from build123d import *

# Parameters (mm, degrees)
SKETCH_1_W      = 85
SKETCH_1_H      = 104
SKETCH_1_R      = 2
SKETCH_1_R_2    = 1.5
EXTRUDE_1_DEPTH = 4
FILLET_1_R      = 8


with BuildPart() as part:
    # 草图1 → 凸台-拉伸1 (new body)
    with BuildSketch(Plane.XY):
        with Locations((-13.600288588, -10.520274333)):
            Rectangle(SKETCH_1_W, SKETCH_1_H)
        with Locations((12.899711412, -0.520274333)):
            Circle(SKETCH_1_R, mode=Mode.SUBTRACT)
        with Locations((12.899711412, -20.520274333)):
            Circle(SKETCH_1_R, mode=Mode.SUBTRACT)
        with Locations((-46.100288588, 14.479725667)):
            Circle(SKETCH_1_R, mode=Mode.SUBTRACT)
        with Locations((-46.100288588, -35.520274333)):
            Circle(SKETCH_1_R, mode=Mode.SUBTRACT)
        with Locations((3.899711412, -35.520274333)):
            Circle(SKETCH_1_R, mode=Mode.SUBTRACT)
        with Locations((3.899711412, 14.479725667)):
            Circle(SKETCH_1_R, mode=Mode.SUBTRACT)
        with Locations((-5.100288588, 31.979725667)):
            Circle(SKETCH_1_R_2, mode=Mode.SUBTRACT)
        with Locations((14.899711412, 31.979725667)):
            Circle(SKETCH_1_R_2, mode=Mode.SUBTRACT)
        with Locations((-5.100288588, -53.020274333)):
            Circle(SKETCH_1_R_2, mode=Mode.SUBTRACT)
        with Locations((14.899711412, -53.020274333)):
            Circle(SKETCH_1_R_2, mode=Mode.SUBTRACT)
    extrude(amount=EXTRUDE_1_DEPTH)

    # 圆角1
    fillet_1_edges = [part.edges().sort_by_distance(p)[0] for p in [
        (28.899711412, -62.520274333, 2),
        (-56.100288588, -62.520274333, 2),
        (-56.100288588, 41.479725667, 2),
        (28.899711412, 41.479725667, 2),
    ]]
    fillet(fillet_1_edges, radius=FILLET_1_R)


solid = part.part
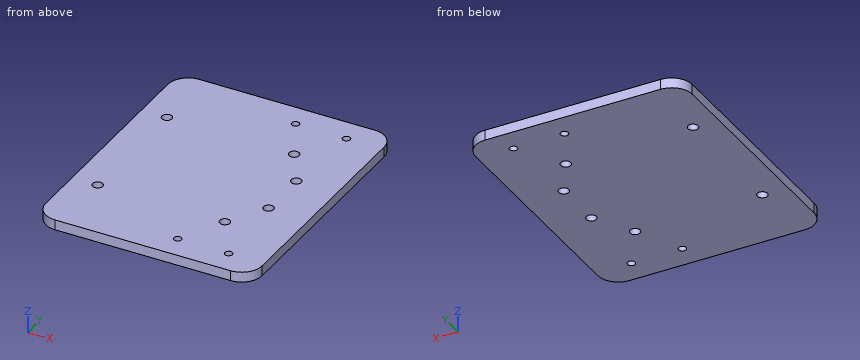
Verification items for the finished model (mm, model axes). Coordinates: 2 decimals unless noted, no trailing zeros. Answer as a JSON object with one key per item and string values.
(1) Thickness scan on line 1 along Y through (x, z) = (-4.5, 2.5); line 2 along X through (y, z) = (36.5, 2.25); line 3 along Y through (x, z) = (-49.5, 3). Record the ranges inside material, lowest first.
Report:
{"line 1": "-62.52 to -54.39, -51.65 to 30.61, 33.35 to 41.48", "line 2": "-55.51 to 28.31", "line 3": "-62.4 to 41.36"}
(2) Gauge pin test, flat end, axial feed: pin 1 Ø5 at (x, y) = (14.9, 31.98) entering from +Z. Record the tip position at first contact, or that the pin passes through.
Report:
{"pin 1": "z = 4"}
(3) Cross-section at A-A on z = 2.85. Give the number of separate pieces and of enclosed holes in the cut face, plus the area to 3 significant figures.
Report:
{"separate pieces": "1", "enclosed holes": "10", "area": "8,680 mm^2"}
